Could you check a few things on this model? Use its own coordinates, in mm. A direction names the side the tool comes from. Coordinates: 2 decimals unless noted, no trailing zeros. Order: outer loops, then holes, each group sorted by start corner. A loop starts at its lowest first (then second) coordinate and runs counter-clockwise, first axis right, second up. Notation, with made-up numbers: (-31.5, 11.5) - (-11.5, 11.5) arc R9 ccw to (-11.5, 19.5) - close; hole circle Ø10 at (82.5, -30). An arc over 180 degrees is marked (long way). One line per item, written item: value.
from build123d import *

# Parameters (mm, degrees)
Y_KSEKLIK_EKSTR_ZYON1_DEPTH = 5
Y_KSEKLIK_EKSTR_ZYON2_DEPTH = 2


with BuildPart() as part:
    # izim1 → Y_kseklik-Ekstr_zyon1 (new body)
    with BuildSketch(Plane(origin=(0, 0, 0), x_dir=(1, 0, 0), z_dir=(0, 1, 0))):
        with BuildLine():
            Line((0, 5), (80, 5))
            ThreePointArc((80, 5), (85, 0), (80, -5))
            Line((80, -5), (0, -5))
            ThreePointArc((0, -5), (-5, 0), (0, 5))
        make_face()
        with BuildLine():
            Line((79.824449331, 3.495594651), (60, 2.5))
            Line((60, 2.5), (60, -2.5))
            Line((60, -2.5), (79.824449331, -3.495594651))
            ThreePointArc((79.824449331, -3.495594651), (83.5, 0), (79.824449331, 3.495594651))
        make_face(mode=Mode.SUBTRACT)
    extrude(amount=Y_KSEKLIK_EKSTR_ZYON1_DEPTH)

    # izim1_4 → Y_kseklik-Ekstr_zyon2 (add)
    with BuildSketch(Plane(origin=(0, 0, 0), x_dir=(1, 0, 0), z_dir=(0, 1, 0))):
        with BuildLine():
            ThreePointArc((79.824449331, -3.495594651), (83.5, 0), (79.824449331, 3.495594651))
            Line((79.824449331, 3.495594651), (60, 2.5))
            Line((60, 2.5), (60, -2.5))
            Line((60, -2.5), (79.824449331, -3.495594651))
        make_face()
    extrude(amount=Y_KSEKLIK_EKSTR_ZYON2_DEPTH)


solid = part.part
Item 1: If I drill on probe 1 along Y at (x, z) = (66, 1); probe 2 along Z at (x, y) = (72, 3.55); probe 3 along X at (y, z) = (3.75, -1.5), over which ranges is the centre line in solid material (lowest first)?
Conclusion:
probe 1: 0 to 2
probe 2: -5 to -3.1, 3.1 to 5
probe 3: -4.77 to 60, 83.16 to 84.77
Item 2: I'm going to push flat-ended pins straight in: pin 1 Ø1.5 at (y, z) = (4, -1) entering from +X; pin 2 Ø1.5 at (y, z) = (0.5, -4) entering from -X; pin 3 Ø3.5 at (x, z) = (68.5, -0.5) entering from +Y. Where does each tip first touch, or does it pass through?
Conclusion:
pin 1: x = 84.99
pin 2: x = -3.8
pin 3: y = 2
Item 3: For faces 4 (the face through (31, 5, 0)), 5 (the face through (72, 2, 0)), which set-ups out of +Z, -Z, +X, -X, +Y, -Y let a thin tool reach every point of the face, with its end or its side?
Conclusion:
face 4: +Z, -Z, +X, -X, +Y
face 5: +Y
Item 4: Thinking about a two-plate mould opening in X: for faces 1 (the face through (39, 2, -5)), 2 (the face through (83.5, 3.5, 0.1)), 3 (the face through (-5, 2, 0)), which applies, pulls with the +X half, pulls with the -X half, needs draft (parallel to the pull), parting line crosses it, or undercut?
Conclusion:
face 1: needs draft
face 2: undercut
face 3: pulls with the -X half
Item 5: I want a section at B-B on z = 0. Please give me the cut outline in (x, y), then the cut area to 4 significant figures.
Conclusion:
outline: (-5, 0) - (85, 0) - (85, 5) - (83.5, 5) - (83.5, 2) - (60, 2) - (60, 5) - (-5, 5) - close
area: 379.5 mm²
Item 6: I want a section at A-A on y = 3.95. Please give me the cut outline in (x, z).
Conclusion:
outline: (0, -5) - (80, -5) arc R5 ccw to (80, 5) - (0, 5) arc R5 ccw to start; hole (60, -2.5) - (79.82, -3.5) arc R3.5 ccw (long way) to (79.82, 3.5) - (60, 2.5) - close
Item 7: I want a section at C-C on x = 75. Please give me the cut outline in (y, z).
Conclusion:
outline: (0, -5) - (5, -5) - (5, -3.25) - (2, -3.25) - (2, 3.25) - (5, 3.25) - (5, 5) - (0, 5) - close
